Autodesk Inventor part; units mm, degrees
ref_plane "YZ Plane" through (0, 0, 0) normal (1, 0, 0) x (0, 1, 0)
ref_plane "XZ Plane" through (0, 0, 0) normal (0, 1, 0) x (-1, 0, 0)
ref_plane "XY Plane" through (0, 0, 0) normal (0, 0, 1) x (1, 0, 0)
sketch "Sketch1" plane through (0, 0, 0) normal (0, 0, 1) x (1, 0, 0)
  line L0 (-12.7, -12.7) -> (12.7, -12.7)
  line L1 (12.7, -12.7) -> (12.7, 12.7)
  line L2 (12.7, 12.7) -> (-12.7, 12.7)
  line L3 (-12.7, 12.7) -> (-12.7, -12.7)
  line L4 (-12.7, -12.7) -> (12.7, 12.7) construction
  line L5 (12.7, -12.7) -> (-12.7, 12.7) construction
  line L6 (-9.525, -9.525) -> (9.525, -9.525)
  line L7 (9.525, -9.525) -> (9.525, 9.525)
  line L8 (9.525, 9.525) -> (-9.525, 9.525)
  line L9 (-9.525, 9.525) -> (-9.525, -9.525)
  line L10 (-9.525, -9.525) -> (9.525, 9.525) construction
  line L11 (9.525, -9.525) -> (-9.525, 9.525) construction
  point P0 (0, 0)
  dimension "d0" = 25.4
  dimension "d1" = 25.4
  dimension "d2" = 3.175
  dimension "d3" = 3.175
extrude "Extrusion1" add sketch "Sketch1" along normal mid plane 254
properties part number "10-inchAluminumTubing"
The listing builds one solid part. Answer for the finished solid, in the listing's coordinates (mm). A direction names the side the tool comes from. Give positions to 0.01 mm unless a question says otherwise; leave off trailing zeros. Write each loop counter-clockwise with the first axis right and the second up, starting at its lowest first coordinate (ties: lowest second). Pieces come first, ordered by that corner, then holes. Notation, with made-up numbers: (4.25, -3.5) -> (29.25, -3.5) arc R17 cw to (29.25, 8.5) -> close; hole circle Ø4 at (22.25, 8). An arc over 180 degrees is marked (long way). Write item = value, one per line. Start each with the question number.
1) A straight line is drawn through the part: line 1 along Y through (x, z) = (-1.5, -52.5) (3 decimals). Find the intervals that lie inside material, in ascending order.
2) The part is cut by section A-A, the plane x = 6.25. Determine the outline of the cut face in (y, z) (3 decimals).
3) Which of the six approach directions +Z, -Z, +X, -X, +Y, -Y give full straight-line access (tool end or side, diameter ignored) to faces 1 (the face through (0, 12.7, -2)), 2 (the face through (0, 9.525, -2))?
4) The part is cut by section B-B, the plane z = 42.5. Determine the outline of the cut face in (x, y) (3 decimals), and give its area (3 significant figures).
5) Determine the mould class of faces 3 (the face through (0, -9.525, -2)), 4 (the face through (11, 0, 127)), 5 (the face through (12.7, 0, -2)), 6 (the face through (-12.7, 0, -2)) for opening direction X: +X half, -X half, draft (parallel to the pull), parting line (faces both ways), or undercut.
Solutions:
q1.line_1 = -12.7 to -9.525, 9.525 to 12.7
q2.outline = (-12.7, -127) -> (-9.525, -127) -> (-9.525, 127) -> (-12.7, 127) -> close; (9.525, -127) -> (12.7, -127) -> (12.7, 127) -> (9.525, 127) -> close
q3.face_1 = +Z, -Z, +X, -X, +Y
q3.face_2 = +Z, -Z
q4.outline = (-12.7, -12.7) -> (12.7, -12.7) -> (12.7, 12.7) -> (-12.7, 12.7) -> close; hole (-9.525, -9.525) -> (9.525, -9.525) -> (9.525, 9.525) -> (-9.525, 9.525) -> close
q4.area = 282 mm²
q5.face_3 = undercut
q5.face_4 = draft
q5.face_5 = +X half
q5.face_6 = -X half
